```python
from build123d import *

# Parameters (mm, degrees)
SKETCH1_R           = 12.4
BOSS_EXTRUDE1_DEPTH = 1.5
SKETCH2_R           = 5
SKETCH2_W           = 0.5
SKETCH2_H           = 4
CUT_EXTRUDE1_DEPTH  = 2.5
FILLET1_R           = 0.05


with BuildPart() as part:
    # Sketch1 → Boss-Extrude1 (new body)
    with BuildSketch(Plane.XY):
        Circle(SKETCH1_R)
    extrude(amount=BOSS_EXTRUDE1_DEPTH)

    # Sketch2 → Cut-Extrude1 (cut, through all)
    with BuildSketch(Plane.XY.offset(1.5)):
        Circle(SKETCH2_R)
        with Locations((-8.7, 0)):
            Rectangle(SKETCH2_W, SKETCH2_H)
        with Locations((8.7, 0)):
            Rectangle(SKETCH2_W, SKETCH2_H)
    extrude(amount=-CUT_EXTRUDE1_DEPTH, mode=Mode.SUBTRACT)

    # Fillet1
    fillet1_edges = [part.edges().sort_by_distance(p)[0] for p in [
        (-8.95, 0, 0),
        (-8.7, 2, 0),
        (-8.45, 0, 0),
        (-8.7, -2, 0),
        (-8.95, 0, 1.5),
        (-8.7, -2, 1.5),
        (-8.45, 0, 1.5),
        (-8.7, 2, 1.5),
        (-12.4, 0, 0),
        (8.45, 0, 0),
        (8.7, 2, 0),
        (8.95, 0, 0),
        (8.7, -2, 0),
        (8.45, 0, 1.5),
        (8.7, -2, 1.5),
        (8.95, 0, 1.5),
        (8.7, 2, 1.5),
        (-12.4, 0, 1.5),
        (-5, 0, 0),
        (-5, 0, 1.5),
    ]]
    fillet(fillet1_edges, radius=FILLET1_R)


solid = part.part
```
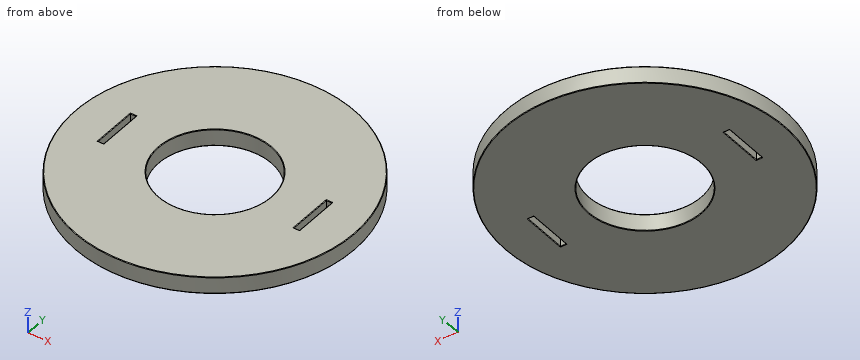
Geometry check sheet. Reference: the model listing, model coordinates, mm. Give positions to 0.01 mm unless a question says otherwise; leave off trailing zeros. Loops run counter-clockwise (first coordinate to the right, second up) from the corner with the lowest first, then second, coordinate; pieces in that order, holes last. Notation, with made-up numbers: (33, 67) - (90, 67) arc R28 cw to (90, 98) - close; hole circle Ø4 at (86.25, 34). An arc over 180 degrees is marked (long way). Use CSV: the item, a comma, the result in double quotes. Start each with the question number.
Q1. Section check C-C, the plane z = 0.35. Record the cut outline in (x, y).
Q2. Section check A-A, the plane y = 0. Count the separate pieces of the cut face and the enclosed holes in it, and give its area (3 significant figures).
Q3. Go/stop test with flat-tipped pins: pin 1 Ø0.6 at (x, z) = (8.5, 0.5) entering from +Y; pin 2 Ø8 at (x, y) = (0, 0) entering from -Z. Record where each tip stops, or that it passes through.
Q4. Scan lines: probe 1 along X at (y, z) = (-1.25, 0.4); probe 2 along Y at (x, z) = (0, 0.85); probe 3 along X at (y, z) = (-3.75, 0.45). Record each from-to range of solid material in increasing order. Write a range as from..to.
Q5. Section check B-B, the plane x = 0. Record the cut outline in (y, z).
Findings below:
1,outline,"circle Ø24.8 at (0, 0); hole (-8.95, -2) - (-8.45, -2) - (-8.45, 2) - (-8.95, 2) - close; hole circle Ø10 at (0, 0); hole (8.45, -2) - (8.95, -2) - (8.95, 2) - (8.45, 2) - close"
2,separate pieces,"4"
2,enclosed holes,"0"
2,area,"20.7 mm^2"
3,pin 1,"stops at y = 9.3"
3,pin 2,"passes through"
4,probe 1,"x = -12.34..-8.95, -8.45..-4.84, 4.84..8.45, 8.95..12.34"
4,probe 2,"y = -12.4..-5, 5..12.4"
4,probe 3,"x = -11.82..-3.31, 3.31..11.82"
5,outline,"(-12.4, 0.05) arc R0.05 ccw to (-12.35, 0) - (-5.05, 0) arc R0.05 ccw to (-5, 0.05) - (-5, 1.45) arc R0.05 ccw to (-5.05, 1.5) - (-12.35, 1.5) arc R0.05 ccw to (-12.4, 1.45) - close; (5, 0.05) arc R0.05 ccw to (5.05, 0) - (12.35, 0) arc R0.05 ccw to (12.4, 0.05) - (12.4, 1.45) arc R0.05 ccw to (12.35, 1.5) - (5.05, 1.5) arc R0.05 ccw to (5, 1.45) - close"
